```python
from build123d import *

# Parameters (mm, degrees)
BOSS_EXTRUDE1_DEPTH = 2
FILLET1_R           = 10
SKETCH3_R           = 1.5
SKETCH3_R_2         = 4
SKETCH3_R_3         = 5
CUT_EXTRUDE1_DEPTH  = 2


with BuildPart() as part:
    # Sketch2 → Boss-Extrude1 (new body)
    with BuildSketch(Plane(origin=(0, 0, 0), x_dir=(1, 0, 0), z_dir=(0, 1, 0))):
        Polygon((0, 0), (65, 165), (-290, 165), (-190, 0), align=None)
    extrude(amount=BOSS_EXTRUDE1_DEPTH)

    # Fillet1
    fillet1_edges = [part.edges().sort_by_distance(p)[0] for p in [
        (-190, 1, 0),
        (-290, 1, -165),
        (65, 1, -165),
        (0, 1, 0),
    ]]
    fillet(fillet1_edges, radius=FILLET1_R)

    # Sketch3 → Cut-Extrude1 (cut)
    with BuildSketch(Plane(origin=(0, 2, 0), x_dir=(1, 0, 0), z_dir=(0, 1, 0))):
        with Locations(Location((-228.170289346, 83, 0), (0, 0, 270))):
            Circle(SKETCH3_R)
        with Locations(Location((-246.246193102, 157, 0), (0, 0, 270))):
            Circle(SKETCH3_R)
        with Locations(Location((-46.246193102, 157, 0), (0, 0, 270))):
            Circle(SKETCH3_R)
        with Locations(Location((11.829710654, 83, 0), (0, 0, 270))):
            Circle(SKETCH3_R)
        with Locations(Location((13.829710654, 144.5, 0), (0, 0, 270))):
            Circle(SKETCH3_R)
        with Locations(Location((27.829710654, 130.5, 0), (0, 0, 270))):
            Circle(SKETCH3_R)
        with Locations(Location((13.829710654, 116.5, 0), (0, 0, 270))):
            Circle(SKETCH3_R)
        with Locations(Location((-0.170289346, 130.5, 0), (0, 0, 270))):
            Circle(SKETCH3_R)
        with Locations(Location((-272.246193102, 155, 0), (0, 0, 90))):
            Circle(SKETCH3_R_2)
        with Locations(Location((-172.246193102, 155, 0), (0, 0, 90))):
            Circle(SKETCH3_R_2)
        with Locations(Location((13.829710654, 130.5, 0), (0, 0, 90))):
            Circle(SKETCH3_R_2)
        with Locations(Location((-236.170289346, 130.5, 0), (0, 0, 90))):
            Circle(SKETCH3_R_2)
        with Locations(Location((-111.170289346, 130.5, 0), (0, 0, 90))):
            Circle(SKETCH3_R_2)
        with Locations(Location((-18.170289346, 83, 0), (0, 0, 90))):
            Circle(SKETCH3_R_3)
        with Locations(Location((-188.170289346, 83, 0), (0, 0, 90))):
            Circle(SKETCH3_R_3)
        with Locations(Location((-98.170289346, 83, 0), (0, 0, 90))):
            Circle(SKETCH3_R_3)
        with Locations(Location((-205.049987171, 40.267503937, 0), (0, 0, 90))):
            Circle(SKETCH3_R)
        with Locations(Location((-208.170289346, 51.5, 0), (0, 0, 90))):
            Circle(SKETCH3_R)
        with Locations(Location((-225.782055815, 74.475417199, 0), (0, 0, 90))):
            Circle(SKETCH3_R)
        with Locations(Location((-236.148090136, 91.57937383, 0), (0, 0, 90))):
            Circle(SKETCH3_R)
        with Locations(Location((-246.514124458, 108.683330462, 0), (0, 0, 90))):
            Circle(SKETCH3_R)
        with Locations(Location((-256.88015878, 125.787287093, 0), (0, 0, 90))):
            Circle(SKETCH3_R)
        with Locations(Location((-267.246193102, 142.891243724, 0), (0, 0, 90))):
            Circle(SKETCH3_R)
        with Locations(Location((1.829710654, 26.47129363, 0), (0, 0, 90))):
            Circle(SKETCH3_R)
        with Locations(Location((9.160201021, 45.079461487, 0), (0, 0, 90))):
            Circle(SKETCH3_R)
        with Locations(Location((16.490691389, 63.687629343, 0), (0, 0, 90))):
            Circle(SKETCH3_R)
        with Locations(Location((23.821181757, 82.295797199, 0), (0, 0, 90))):
            Circle(SKETCH3_R)
        with Locations(Location((31.151672124, 100.903965056, 0), (0, 0, 90))):
            Circle(SKETCH3_R)
        with Locations(Location((38.482162492, 119.512132912, 0), (0, 0, 90))):
            Circle(SKETCH3_R)
        with Locations(Location((-72.246193102, 155, 0), (0, 0, 90))):
            Circle(SKETCH3_R_2)
        with Locations(Location((-148.170289346, 154.5, 0), (0, 0, 90))):
            Circle(SKETCH3_R)
        with Locations(Location((-188.170289346, 114.5, 0), (0, 0, 90))):
            Circle(SKETCH3_R)
        with Locations(Location((-148.170289346, 114.5, 0), (0, 0, 90))):
            Circle(SKETCH3_R)
        with Locations(Location((-108.170289346, 114.5, 0), (0, 0, 90))):
            Circle(SKETCH3_R)
        with Locations(Location((-68.170289346, 114.5, 0), (0, 0, 90))):
            Circle(SKETCH3_R)
        with Locations(Location((-28.170289346, 114.5, 0), (0, 0, 90))):
            Circle(SKETCH3_R)
        with Locations(Location((-148.170289346, 83, 0), (0, 0, 90))):
            Circle(SKETCH3_R)
        with Locations(Location((-215.416021493, 57.371460568, 0), (0, 0, 90))):
            Circle(SKETCH3_R)
        with Locations(Location((-168.170289346, 51.5, 0), (0, 0, 90))):
            Circle(SKETCH3_R)
        with Locations(Location((-8.170289346, 51.5, 0), (0, 0, 90))):
            Circle(SKETCH3_R)
        with Locations(Location((-128.170289346, 51.5, 0), (0, 0, 90))):
            Circle(SKETCH3_R)
        with Locations(Location((-88.170289346, 51.5, 0), (0, 0, 90))):
            Circle(SKETCH3_R)
        with Locations(Location((-48.170289346, 83, 0), (0, 0, 90))):
            Circle(SKETCH3_R)
        with Locations(Location((-48.170289346, 51.5, 0), (0, 0, 90))):
            Circle(SKETCH3_R)
        with Locations(Location((-8.170289346, 12, 0), (0, 0, 90))):
            Circle(SKETCH3_R_2)
        with Locations(Location((-148.170289346, 20, 0), (0, 0, 90))):
            Circle(SKETCH3_R)
        with Locations(Location((-98.170289346, 12, 0), (0, 0, 90))):
            Circle(SKETCH3_R_2)
        with Locations(Location((-48.170289346, 20, 0), (0, 0, 90))):
            Circle(SKETCH3_R)
    extrude(amount=-CUT_EXTRUDE1_DEPTH, mode=Mode.SUBTRACT)


solid = part.part
```
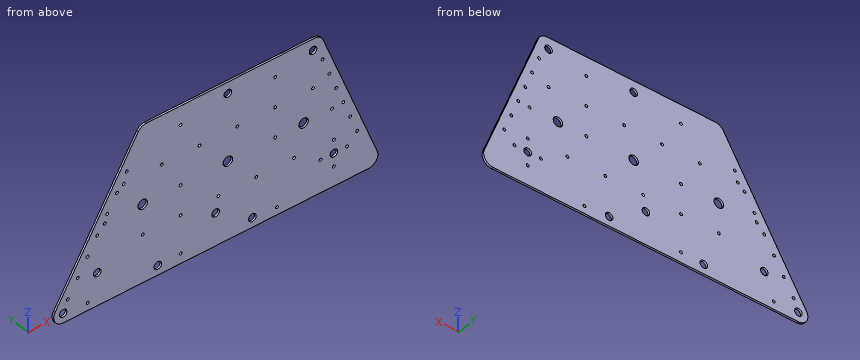
CAD build for the part. Positions are in the model's coordinates, mm. Coordinates: 2 decimals unless noted, no trailing zeros. Order: outer loops, then holes, each group sorted by start corner. A loop starts at its lowest first (then second) coordinate and runs counter-clockwise, first axis right, second up. Notation, with made-up numbers: (-11.75, 59.5) - (31.25, 59.5) arc R32 cw to (31.25, 93.5) - close; hole circle Ø10 at (-0.5, 3.25). An arc over 180 degrees is marked (long way). Use a Markdown table: item, result. Add a question column.
(1) Drill centre lines: line 1 along X through (y, z) = (1.45, -155); line 2 along Z through (x, y) = (-147, 0.2); line 3 along Z through (x, y) = (-47, 0.95). Where is each one in solid material? Low to high. Write a range as [from, to].
(2) Saw through at B-B (z = -31.5). Give the cut face in (x, y).
(3) Saw through at A-A (y = 1.55). Count the separate pieces of the cut face and the enclosed holes in it, then the cut area to 3 significant figures.
Solved:
| question | item | result |
|---|---|---|
| 1 | line 1 | x = [-282.25, -276.25], [-268.25, -176.25], [-168.25, -149.58], [-146.76, -76.25], [-68.25, 60.31] |
| 1 | line 2 | z = [-165, -155.44], [-153.56, -115.44], [-113.56, -83.94], [-82.06, -20.94], [-19.06, 0] |
| 1 | line 3 | z = [-165, -158.3], [-155.7, -83.94], [-82.06, -52.44], [-50.56, -20.94], [-19.06, 0] |
| 2 | outline | (-209.09, 0) - (12.41, 0) - (12.41, 2) - (-209.09, 2) - close |
| 3 | separate pieces | 1 |
| 3 | enclosed holes | 48 |
| 3 | area | 43,900 mm² |
